Verification items for this drawing (mm, ordinates from the low corner). A direction names the side the tool comes from. Coordinates: 2 decimals unless noted, no trailing zeros. Loops run counter-clockwise (first coordinate to the right, second up) from the corner with the lowest first, then second, coordinate; pieces in that order, holes last. Notation, with made-up numbers: (65, -29.75) - (84, -29.75) arc R23 ccw to (84, -3.75) - close; hole circle Ø8 at (74.25, 15). An arc over 180 degrees is marked (long way). One line per item, written item: value. Start each with the question number.
(1) Section check A-A (x = 20). Record the boundary of the cut face in (y, z).
(2) Section check B-B (y = 20). Record the boundary of the cut face in (x, z).
(3) Thickness scan on probe 1 along X at (y, z) = (20, 8.25); probe 2 along Y at (x, z) = (16, 4.75). Record the ranges inside material, lowest first. Write a range as [from, to].
(4) Gauge pin test, flat ends, axial feed: P1, Ø0.9, axis at x = 37, z = 19, coming from the +Y side; P2, Ø1, axis at y = 7, z = 5, coming from the +X side; P3, Ø5, axis at x = 30, z = 5.5, coming from the +Y side. Record the tip position at first contact, or that the pin passes through.
(5) Section check C-C (z = 16.5). Record the boundary of the cut face in (x, y).
(6) Set-up check for the marked faces 1 and 2: record each of +Z, -Z, +X, -X, +Y, -Y from which the full face is reachable in a straight line by a thin tool's end or side.
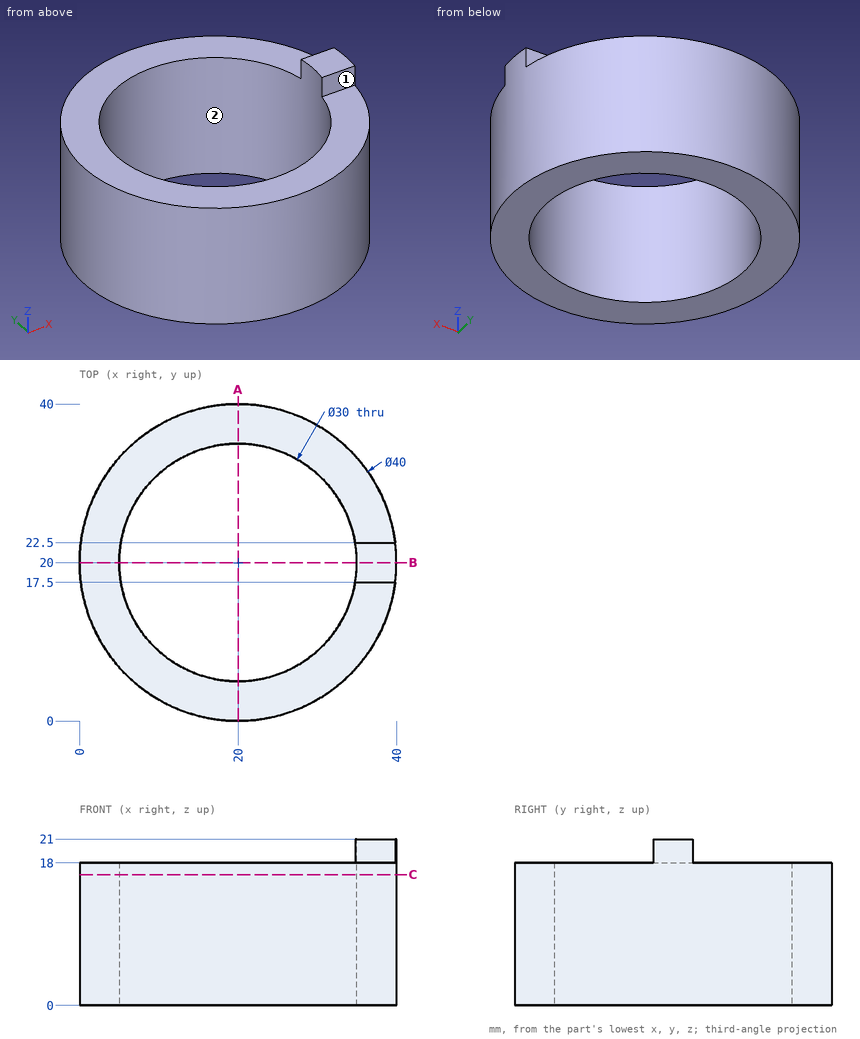
Responses:
1. outline: (0, 0) - (5, 0) - (5, 18) - (0, 18) - close; (35, 0) - (40, 0) - (40, 18) - (35, 18) - close
2. outline: (0, 0) - (5, 0) - (5, 18) - (0, 18) - close; (35, 0) - (40, 0) - (40, 21) - (35, 21) - close
3. probe 1: x = [0, 5], [35, 40]
3. probe 2: y = [0.4, 5.54], [34.46, 39.6]
4. P1: stops at y = 22.5
4. P2: stops at x = 35.61
4. P3: stops at y = 38.54
5. outline: circle Ø40 at (20, 20); hole circle Ø30 at (20, 20)
6. face 1: +Z, +X, -X, -Y
6. face 2: +Z, -Z
